Build history of the part. All positions in model axes, mm. A direction names the side the tool comes from. Round coordinates to 2 decimals unless told otherwise and drop trailing zeros. Order: outer loops, then holes, each group sorted by start corner. A loop starts at its lowest first (then second) coordinate and runs counter-clockwise, first axis right, second up. Notation, with made-up numbers: M 88.5,-8 L 107.5,-8 A31 ccw 107.5,30 Z; hole C -6.75,-13.75 d10. An arc over 180 degrees is marked long. One line per item, written item: value. Start each with the question number.
Item 1: Band-saw the part on A-A, the plane y = -9. Write the cut outline in (x, z).
Item 2: Band-saw the part on B-B, the plane x = 0. Write the cut outline in (y, z), then the cut area to 3 significant figures.
Item 3: Pin check, flat tips, straight feed: pin 1 (3 mm diameter, centred on x = 1, z = -19, fed in from +Y); pin 2 (2 mm diameter, centred on x = 1, z = -3.5, fed in from -Y); pin 3 (2.5 mm diameter, centred on x = -1.5, y = 10.5, fed in from -Z). Stop position of each tip, or through.
Item 4: Band-saw the part on C-C, the plane z = -16. Write the cut outline in (x, y).
Item 5: Two-plate mould, pull along Z, no slides. Class faces 6 (the flat face through (0, -7, 0)), 7 (the flat face through (0, 13, 2)), 8 (the flat face through (0, 0, 4)), 9 (the cylindrical face through (0, 0, -13)): +Z half, -Z half, draft (parallel to the pull), parting line (faces both ways), or undercut.
Item 6: Band-saw the part on D-D, the plane y = 0. Write the cut outline in (x, z).
Item 7: Probe L1, parallel to X at y = 0, z = -21.3; L2, parallel to Y at x = 0, z = 1.85; L3, parallel to Y at x = 0, z = -21.1. List the from-to ranges inside material, lowest first.
Item 8: Tool access for faces 1 (the flat face through (0, 5, -12)), 2 (the flat face through (0, -5, -12)), 3 (the cylindrical face through (0.228, -7.265, 1.972)), 4 (the flat face through (0, -13, 2)), 5 (the cylindrical face through (0.228, 1.735, -21.257)): list every direction of +Z, -Z, +X, -X, +Y, -Y with a clear straight run to the whole face (end or side of a thin tool).
```python
from build123d import *

# Parameters (mm, degrees)
SKETCH1_W               = 8
SKETCH1_H               = 26
BOSS_EXTRUDE1_DEPTH     = 4
SKETCH2_R               = 1.75
CUT_EXTRUDE1_DEPTH      = 4
SKETCH3_W               = 8
SKETCH3_H               = 10
BOSS_EXTRUDE2_DEPTH     = 24
SKETCH4_R               = 3
CUT_EXTRUDE2_DEPTH      = 20
CUT_EXTRUDE3_REACH      = 33.129
CUT_EXTRUDE3_END_RADIUS = 3
SKETCH5_R               = 1.75


with BuildPart() as part:
    # Sketch1 → Boss-Extrude1 (new body)
    with BuildSketch(Plane.XY):
        Rectangle(SKETCH1_W, SKETCH1_H)
    extrude(amount=BOSS_EXTRUDE1_DEPTH)

    # Sketch2 → Cut-Extrude1 (cut)
    with BuildSketch(Plane(origin=(0, 0, 0), x_dir=(-1, 0, 0), z_dir=(0, 0, -1))):
        with Locations((0, 9)):
            Circle(SKETCH2_R)
        with Locations((0, -9)):
            Circle(SKETCH2_R)
    extrude(amount=-CUT_EXTRUDE1_DEPTH, mode=Mode.SUBTRACT)

    # Sketch3 → Boss-Extrude2 (add)
    with BuildSketch(Plane(origin=(0, 0, 0), x_dir=(-1, 0, 0), z_dir=(0, 0, -1))):
        Rectangle(SKETCH3_W, SKETCH3_H)
    extrude(amount=BOSS_EXTRUDE2_DEPTH)

    # Sketch4 → Cut-Extrude2 (cut)
    with BuildSketch(Plane(origin=(4, 0, 0), x_dir=(0, 0, -1), z_dir=(1, 0, 0))):
        with Locations(Location((16, 0, 0), (0, 0, 90))):
            Circle(SKETCH4_R)
    extrude(amount=-CUT_EXTRUDE2_DEPTH, mode=Mode.SUBTRACT)

    # Cut-Extrude3: up to this cylinder (the profile starts outside it)
    cut_extrude3_end = Plane(origin=(0, 0, -16), z_dir=(1, 0, 0)) * Cylinder(CUT_EXTRUDE3_END_RADIUS, 73.258, mode=Mode.PRIVATE)
    # Sketch5 → Cut-Extrude3 (cut, up to the surface)
    with BuildSketch(Plane(origin=(0, 0, -24), x_dir=(-1, 0, 0), z_dir=(0, 0, -1)), mode=Mode.PRIVATE) as cut_extrude3_sk1:
        Circle(SKETCH5_R)
    cut_extrude3_tool1 = extrude(cut_extrude3_sk1.sketch, amount=-CUT_EXTRUDE3_REACH, mode=Mode.PRIVATE) - cut_extrude3_end
    add(cut_extrude3_tool1.solids().sort_by_distance((0, 0, -24))[0], mode=Mode.SUBTRACT)


solid = part.part
```
Output:
1. outline: M -4,0 L -1.75,0 L -1.75,4 L -4,4 Z; M 1.75,0 L 4,0 L 4,4 L 1.75,4 Z
2. outline: M -13,0 L -10.75,0 L -10.75,4 L -13,4 Z; M -7.25,0 L -5,0 L -5,-24 L -1.75,-24 L -1.75,-18.44 A3 cw long 1.75,-18.44 L 1.75,-24 L 5,-24 L 5,0 L 7.25,0 L 7.25,4 L -7.25,4 Z; M 10.75,0 L 13,0 L 13,4 L 10.75,4 Z
2. area: 270 mm²
3. pin 1: stops at y = 5
3. pin 2: stops at y = -5
3. pin 3: stops at z = 0
4. outline: M -4,-5 L 4,-5 L 4,-3 L -4,-3 Z; M -4,3 L 4,3 L 4,5 L -4,5 Z
5. face 6: -Z half
5. face 7: draft
5. face 8: +Z half
5. face 9: undercut
6. outline: M -4,-24 L -1.75,-24 L -1.75,-19 L -4,-19 Z; M -4,-13 L 4,-13 L 4,4 L -4,4 Z; M 1.75,-24 L 4,-24 L 4,-19 L 1.75,-19 Z
7. L1: x = -4 to -1.75, 1.75 to 4
7. L2: y = -13 to -10.75, -7.25 to 7.25, 10.75 to 13
7. L3: y = -5 to -1.75, 1.75 to 5
8. face 1: -Z, +X, -X, +Y
8. face 2: -Z, +X, -X, -Y
8. face 3: +Z, -Z
8. face 4: +Z, -Z, +X, -X, -Y
8. face 5: -Z
